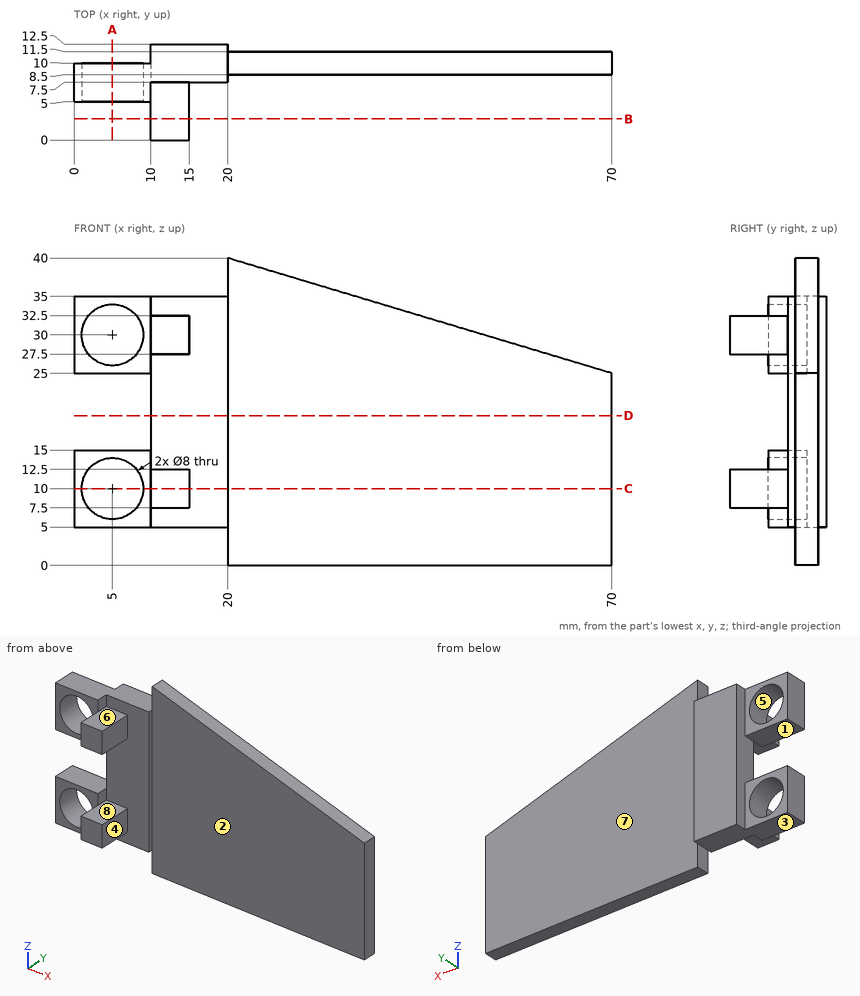
Geometry: see drawing. Coordinates: mm, zero at the bounding-box minimum. A direction names the side the tool comes from. Coordinates: 2 decimals unless noted, no trailing zeros. Write each loop counter-clockwise with the first axis right and the second up, starting at its lowest first coordinate (ties: lowest second). Pieces come first, ordered by that corner, then holes.
1) Mould query, pull axis Z, two halves, no side actions, for the marked faces 1, 2 and 3. Classes: pulls with the +Z half, pulls with the -Z half, needs draft (parallel to the pull), parting line crosses it, or undercut.
2) Section A-A on x = 5. Output: boundary loops of the cut face in (y, z), and give its area (3 significant figures).
3) Section C-C on z = 10. Output: boundary loops of the cut face in (x, y).
4) Section D-D on z = 19.5. Output: boundary loops of the cut face in (x, y).
5) Material intervals for line 1 along X through (y, z) = (6.55, 30); line 2 along X through (y, z) = (7.95, 10); line 3 along Y through (x, z) = (46.5, 7.5), sorted ascending.
6) Pin query (flat end, axial travel): pin 1 Ø12 at (x, z) = (55, 32) entering from -Y; pin 2 Ø2.5 at (x, y) = (13, 2.5) entering from +Z; pin 3 Ø5.5 at (x, y) = (3.5, 8) entering from +Z. Return the tip coordinate at first contact, or that it passes through.
7) Set-up query: the marked faces 4, 5, 6, 7 and 8. Return all of +Z, -Z, +X, -X, +Y, -Y with unobstructed straight access to the full face (end or side cutting, diameter ignored); none if empty.
8) Section B-B on y = 2.75. Output: boundary loops of the cut face in (x, z).
Check result:
1. face 1: undercut
1. face 2: needs draft
1. face 3: pulls with the -Z half
2. outline: (5, 5) - (10, 5) - (10, 6) - (5, 6) - close; (5, 14) - (10, 14) - (10, 15) - (5, 15) - close; (5, 25) - (10, 25) - (10, 26) - (5, 26) - close; (5, 34) - (10, 34) - (10, 35) - (5, 35) - close
2. area: 20.0 mm2
3. outline: (0, 5) - (1, 5) - (1, 10) - (0, 10) - close; (9, 5) - (10, 5) - (10, 0) - (15, 0) - (15, 7.5) - (20, 7.5) - (20, 8.5) - (70, 8.5) - (70, 11.5) - (20, 11.5) - (20, 12.5) - (10, 12.5) - (10, 10) - (9, 10) - close
4. outline: (10, 7.5) - (20, 7.5) - (20, 8.5) - (70, 8.5) - (70, 11.5) - (20, 11.5) - (20, 12.5) - (10, 12.5) - close
5. line 1: x = 0 to 1, 9 to 15
5. line 2: x = 0 to 1, 9 to 20
5. line 3: y = 8.5 to 11.5
6. pin 1: stops at y = 8.5
6. pin 2: stops at z = 32.5
6. pin 3: stops at z = 35
7. face 4: +Z, -Z, +X, -Y
7. face 5: +Y, -Y
7. face 6: +Z, +X, -Y
7. face 7: +Z, -Z, +X, +Y
7. face 8: +X, -Y
8. outline: (10, 7.5) - (15, 7.5) - (15, 12.5) - (10, 12.5) - close; (10, 27.5) - (15, 27.5) - (15, 32.5) - (10, 32.5) - close
